Geometry: final body of the model. Coordinates: model frame, mm. Face numbers are marked on the shaded views. A direction names the side the tool comes from. Round coordinates to 2 decimals unless told otherwise and drop trailing zeros. Loops run counter-clockwise (first coordinate to the right, second up) from the corner with the lowest first, then second, coordinate; pieces in that order, holes last. Notation, with made-up numbers: M 61.5,-30.5 L 113.5,-30.5 A18 cw 113.5,-16.5 Z; hole C -28.5,-8.5 d3. An arc over 180 degrees is marked long. Write each question's results on one line, items separated by ' | '.
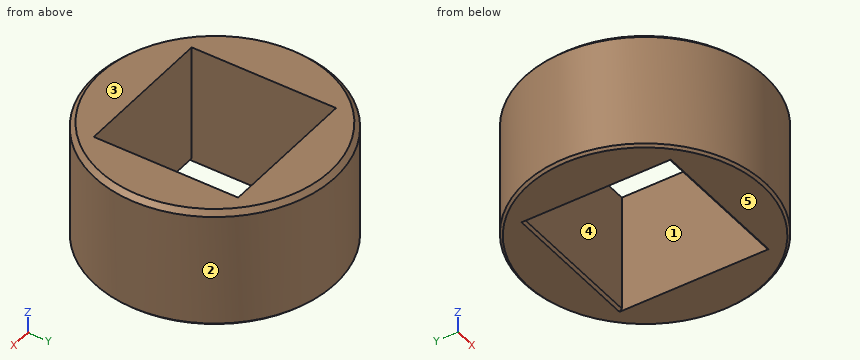
```python
from build123d import *

# Parameters (mm, degrees)
BOX717_W           = 30.2
BOX717_H           = 30.2
BOX717_DEPTH       = 25
CYLINDER1805_R     = 25.15
CYLINDER1805_DEPTH = 25
CHAMFER067_SIZE    = 0.5
CHAMFER066_SIZE    = 1
CHAMFER068_SIZE    = 0.5


with BuildPart() as krychle717:
    # Box717 → Box717 (new body)
    with BuildSketch(Plane(origin=(-15.1, -15.1, 0), x_dir=(1, 0, 0), z_dir=(0, 0, 1))):
        with Locations((15.1, 15.1)):
            Rectangle(BOX717_W, BOX717_H)
    extrude(amount=BOX717_DEPTH)


with BuildPart() as chamfer068:
    # Cylinder1805 → Cylinder1805 (new body)
    with BuildSketch(Plane.XY):
        Circle(CYLINDER1805_R)
    extrude(amount=CYLINDER1805_DEPTH)

    # Cut531: cut Krychle717
    add(krychle717.part, mode=Mode.SUBTRACT)

    # Chamfer067
    chamfer067_edges = [chamfer068.edges().sort_by_distance(p)[0] for p in [
        (0, -15.1, 0),
        (0, 15.1, 0),
    ]]
    chamfer(chamfer067_edges, length=CHAMFER067_SIZE)

    # Chamfer066
    chamfer066_edges = [chamfer068.edges().sort_by_distance(p)[0] for p in [
        (-25.15, 0, 25),
    ]]
    chamfer(chamfer066_edges, length=CHAMFER066_SIZE)

    # Chamfer068
    chamfer068_edges = [chamfer068.edges().sort_by_distance(p)[0] for p in [
        (-25.15, 0, 0),
    ]]
    chamfer(chamfer068_edges, length=CHAMFER068_SIZE)


solid = chamfer068.part
```
1. Pin query (flat end, axial travel): P1, Ø6, axis at x = 11.5, z = 22.5, coming from the +Y side; P2, Ø1.5, axis at y = 6.5, z = 21, coming from the +X side; P3, Ø12, axis at x = 3, z = 7, coming from the -Y side. Return the tip coordinate at first contact, or that it passes through.
Answer key:
P1: stops at y = 23.67 | P2: stops at x = 24.48 | P3: stops at y = -25.15
2. Ray query, probe 1 along X at (y, z) = (5, 9.75); probe 2 along X at (y, z) = (-7.5, 3.75); probe 3 along Y at (x, z) = (-6, 21.25). Return the intervals inside material, ascending.
Answer key:
probe 1: x = -24.65 to -15.1, 15.1 to 24.65 | probe 2: x = -24.01 to -15.1, 15.1 to 24.01 | probe 3: y = -24.42 to -15.1, 15.1 to 24.42
3. Section B-B (y = 0). Output: boundary loops of the cut face in (x, z).
Answer key:
outline: M -25.15,0.5 L -24.65,0 L -15.1,0 L -15.1,25 L -24.15,25 L -25.15,24 Z; M 15.1,0 L 24.65,0 L 25.15,0.5 L 25.15,24 L 24.15,25 L 15.1,25 Z
4. Section C-C (z = 3). Output: boundary loops of the cut face in (x, y).
Answer key:
outline: C 0,0 d50.3; hole M -15.1,-15.1 L 15.1,-15.1 L 15.1,15.1 L -15.1,15.1 Z
5. Draft query along X for the marked faces 1, 2 and 3. Return one class per face: pulls with the +X half, pulls with the -X half, needs draft (parallel to the pull), parting line crosses it, or undercut.
Answer key:
face 1: undercut | face 2: parting line crosses it | face 3: needs draft
6. Section A-A (x = 0). Output: boundary loops of the cut face in (y, z).
Answer key:
outline: M -25.15,0.5 L -24.65,0 L -15.6,0 L -15.1,0.5 L -15.1,25 L -24.15,25 L -25.15,24 Z; M 15.1,0.5 L 15.6,0 L 24.65,0 L 25.15,0.5 L 25.15,24 L 24.15,25 L 15.1,25 Z
7. Access query for the marked faces 4 and 5. Directions: +Z, -Z, +X, -X, +Y, -Y. A direction counts if a zero-diameter tool reaches every point of the face in a straight line with its end or side. Return the directions, or none.
Answer key:
face 4: +Z, -Z | face 5: -Z, +X, -X, +Y, -Y
